CAD build for the part. Positions are in the model's coordinates, mm. Face numbers are marked on the shaded views. A direction names the side the tool comes from. Round coordinates to 2 decimals unless told otherwise and drop trailing zeros. Write each loop counter-clockwise with the first axis right and the second up, starting at its lowest first coordinate (ties: lowest second). Pieces come first, ordered by that corner, then holes. Notation, with made-up numbers: (66.25, 61.25) - (92.25, 61.25) arc R15 ccw to (92.25, 73.25) - close; hole circle Ø8 at (21.5, 3.25). An arc over 180 degrees is marked (long way). Answer in a Markdown table with one row per item.
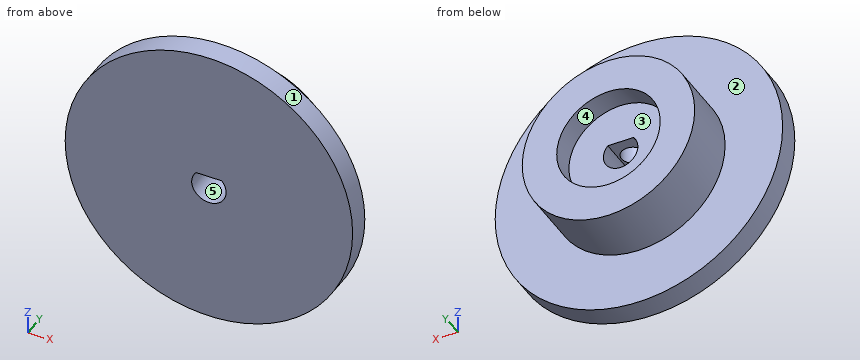
Autodesk Inventor part; units mm, degrees
ref_plane "YZ Plane" through (0, 0, 0) normal (1, 0, 0) x (0, 1, 0)
ref_plane "XZ Plane" through (0, 0, 0) normal (0, 1, 0) x (-1, 0, 0)
ref_plane "XY Plane" through (0, 0, 0) normal (0, 0, 1) x (1, 0, 0)
sketch "Esquisse3" plane through (0, 0, 0) normal (0, 1, 0) x (-1, 0, 0)
  circle A0 centre (0, 0) radius 12.5
  dimension "d3" = 25
extrude "Extrusion2" add sketch "Esquisse3" along normal blind 2
sketch "Esquisse4" plane through (0, 2, 0) normal (0, 1, 0) x (1, 0, 0)
  circle A0 centre (0, 0) radius 12.5
  circle A1 centre (0, 0) radius 7.5
  dimension "d6" = 15
extrude "Extrusion3" add sketch "Esquisse4" along normal blind 5 contours A1
sketch "Esquisse5" plane through (0, 7, 0) normal (0, 1, 0) x (1, 0, 0)
  circle A0 centre (0, 0) radius 7.5
  circle A1 centre (0, 0) radius 4.5
  dimension "d9" = 9
extrude "Extrusion4" cut sketch "Esquisse5" against normal blind 2 contours A1
sketch "Esquisse6" plane through (0, 5, 0) normal (0, 1, 0) x (1, 0, 0)
  circle A0 centre (0, 0) radius 4.5
  circle A1 centre (0, 0) radius 1.5
  line L0 (-1.118, -1) -> (1.118, -1)
  dimension "d12" = 3
  dimension "d13" = 2.5
extrude "Extrusion5" cut sketch "Esquisse6" against normal through all contours A1 L0 picked at (0.0594, -0.1702)
hole "Perçage1" at (-0.041, 3.0497, 1) direction (0, 0, 1) diameter 2 end through all
properties part number "Poulie1"
Q1. Saw through at A-A on z = 0. List the corners of the cut face in (x, y), then the cut area to 3 significant figures.
Computed:
| item | result |
|---|---|
| outline | (-12.5, 0) - (-1.5, 0) - (-1.5, 5) - (-4.5, 5) - (-4.5, 7) - (-7.5, 7) - (-7.5, 2) - (-12.5, 2) - close; (1.5, 0) - (12.5, 0) - (12.5, 2) - (7.5, 2) - (7.5, 7) - (4.5, 7) - (4.5, 5) - (1.5, 5) - close |
| area | 92.0 mm2 |
Q2. Saw through at C-C on y = 5.5. List the corners of the cut face in (x, z).
Computed:
| item | result |
|---|---|
| outline | circle Ø15 at (0, 0); hole circle Ø9 at (0, 0) |
Q3. Pull direction Z, two halves, no side cores. Call the marked faces 1, 2 and 3: released by +Z, released by -Z, zero draft, split by the parting line, or undercut.
Computed:
| item | result |
|---|---|
| face 1 | split by the parting line |
| face 2 | zero draft |
| face 3 | undercut |
Q4. Drill centre lines: line 1 (Z direction, x = 0, y = 1.1); line 2 (X direction, y = 3.8, z = 0); line 3 (Z direction, x = 0, y = 6.05). Where is each one in solid material? Low to high.
Computed:
| item | result |
|---|---|
| line 1 | z = -12.5 to -1.5, 1 to 12.5 |
| line 2 | x = -7.5 to -1.5, 1.5 to 7.5 |
| line 3 | z = -7.5 to -4.5, 4.5 to 7.5 |
Q5. 3-axis set-ups, long thin cutter, end or side, ignore diameter. For the marked faces 4 and 5: which of +Z, -Z, +X, -X, +Y, -Y reach the whole face in a straight line?
Computed:
| item | result |
|---|---|
| face 4 | +Y |
| face 5 | +Y, -Y |
Q6. Flat gauge pins, fed straight in: pin 1 (1.8 mm diameter, centred on x = -0.04, y = 3.05, fed in from +Z); pin 2 (1.1 mm diameter, centred on x = 0, y = 3, fed in from -Z); pin 3 (4 mm diameter, centred on x = 5.5, y = 2.5, fed in from -Z). Where does each tip first touch, or does it go through?
Computed:
| item | result |
|---|---|
| pin 1 | stops at z = -1.17 |
| pin 2 | stops at z = -7.5 |
| pin 3 | stops at z = -11.98 |
Q7. Saw through at B-B on z = 2.75. List the corners of the cut face in (x, y), then the cut area to 3 significant figures.
Computed:
| item | result |
|---|---|
| outline | (-12.19, 0) - (12.19, 0) - (12.19, 2) - (6.98, 2) - (6.98, 7) - (3.56, 7) - (3.56, 5) - (-3.56, 5) - (-3.56, 7) - (-6.98, 7) - (-6.98, 2) - (-12.19, 2) - close; hole circle Ø2 at (-0.04, 3.05) |
| area | 101 mm2 |
Q8. Saw through at D-D on z = -6.75. List the corners of the cut face in (x, y), then the cut area to 3 significant figures.
Computed:
| item | result |
|---|---|
| outline | (-10.52, 0) - (10.52, 0) - (10.52, 2) - (3.27, 2) - (3.27, 7) - (-3.27, 7) - (-3.27, 2) - (-10.52, 2) - close |
| area | 74.8 mm2 |
